Autodesk Fusion 360 part; units mm, degrees
sketch "Sketch1" plane through (0, 0, 0) normal (0, 0, 1) x (1, 0, 0)
  line L0 (0, 0) -> (20, 0)
  line L1 (20, 90) -> (0, 90)
  line L2 (0, 90) -> (0, 0)
  line L3 (4, 79) -> (11.125, 79)
  line L4 (11.125, 79) -> (11.125, 84)
  line L5 (4, 11) -> (4, 79)
  line L6 (0, 75) -> (0, 25)
  line L7 (20, 90) -> (0, 0) construction
  line L8 (0, 90) -> (20, 0) construction
  line L9 (0, 90) -> (-23, 90)
  line L10 (-23, 90) -> (-23, 0)
  line L11 (-23, 0) -> (0, 0)
  line L12 (0, 0) -> (0, 90)
  line L13 (0, 90) -> (-23, 0) construction
  line L14 (-23, 90) -> (0, 0) construction
  line L15 (10, 45) -> (-11.5, 45) construction
  line L16 (0, 86) -> (-19, 86)
  line L17 (-19, 86) -> (-19, 4)
  line L18 (-19, 4) -> (0, 4)
  line L19 (12, 90) -> (12, 0) construction
  line L20 (11.125, 84) -> (12, 84)
  line L21 (20, 79) -> (12.875, 79)
  line L22 (12.875, 79) -> (12.875, 84)
  line L23 (12.875, 84) -> (12, 84)
  line L24 (20, 90) -> (20, 0)
  line L25 (20, 11) -> (12.875, 11)
  line L26 (4, 11) -> (11.125, 11)
  line L27 (11.125, 11) -> (11.125, 6)
  line L28 (11.125, 6) -> (12, 6)
  line L29 (12.875, 6) -> (12, 6)
  line L30 (12.875, 11) -> (12.875, 6)
  point P0 (-11.5, 45)
  dimension "d37" = 90
  dimension "d38" = 23
  dimension "d39" = -4
  dimension "d51" = 12
  dimension "d57" = 1.75
  dimension "d63" = 5
  dimension "d65" = 78
  dimension "d66" = 6
  dimension "d67" = 20
  dimension "d72" = 8
extrude "Extrude7" add sketch "Sketch1" along normal blind 5 contours L2 L6 L12 L16 L17 L18 | L3 L4 L5 L20 L21 L22 L23 L24 L25 L26 L27 L28 L29 L30 makes body 1 at (6.375, 33.6667, 0) makes body 2 at (-6.3333, 58.6667, 0)
extrude "Extrude9" add sketch "Sketch1" along normal blind 70 contours L0 L1 L2 L3 L4 L5 L6 L12 L20 L21 L22 L23 L24 L25 L26 L27 L28 L29 L30 bodies 1 2
extrude "Extrude10" add sketch "Sketch1" along normal blind 100 contours L2 L9 L10 L11 L12 L16 L17 L18 bodies 1
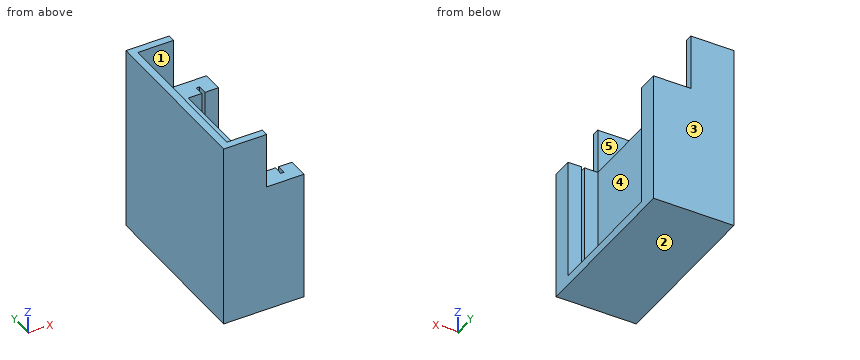
Geometry: final body of the model. Coordinates: model frame, mm. Face numbers are marked on the shaded views. A direction names the side the tool comes from. Round coordinates to 2 decimals unless told otherwise and drop trailing zeros. Loops run counter-clockwise (first coordinate to the right, second up) from the corner with the lowest first, then second, coordinate; pieces in that order, holes last. Notation, with made-up numbers: (-12.75, 59) -> (-1.75, 59) arc R30 cw to (-1.75, 90) -> close; hole circle Ø9 at (11.5, 79.5). An arc over 180 degrees is marked (long way). Use one line per item in the form item = value. Start each with the question number.
1) Section B-B on z = 72. Output: boundary loops of the cut face in (x, y), then the cut area to 3 significant figures.
2) Section A-A on z = 55. Output: boundary loops of the cut face in (x, y) (3 decimals).
3) Section C-C on y = 39.5. Output: boundary loops of the cut face in (x, z), then the cut area to 3 significant figures.
4) First-contact query: P1, Ø4, axis at x = 2.5, z = 76.5, coming from the -Y side; P2, Ø1, axis at y = 70.5, z = 73.5, coming from the +X side; P3, Ø3, axis at y = 2.5, z = 92.5, coming from the +X side; P4, Ø4, axis at y = 70, z = 26, coming from the +X side. Flat tips, straight axial feed; report the tip coordinate or a pass-through.
5) Draft query along X for the marked faces 3, 4 and 5. Return one class per face: released by +X, released by -X, zero draft, split by the parting line, or undercut.
6) Section D-D on x = -10. Output: boundary loops of the cut face in (y, z).
7) Access query for the marked faces 1 and 2. Directions: +Z, -Z, +X, -X, +Y, -Y. A direction counts if a zero-diameter tool reaches every point of the face in a straight line with its end or side. Return the directions, or none.
8) Line query: L1, parallel to X at y = 25.5, z = 60; L2, parallel to Y at x = -18, z = 63.5; L3, parallel to X at y = 7, z = 20 (3 decimals). Output: solid intervals per line, ascending.
Response:
q1.outline = (-23, 0) -> (0, 0) -> (0, 4) -> (-19, 4) -> (-19, 86) -> (0, 86) -> (0, 90) -> (-23, 90) -> close
q1.area = 512 mm^2
q2.outline = (-23, 0) -> (20, 0) -> (20, 11) -> (12.875, 11) -> (12.875, 6) -> (11.125, 6) -> (11.125, 11) -> (4, 11) -> (4, 79) -> (11.125, 79) -> (11.125, 84) -> (12.875, 84) -> (12.875, 79) -> (20, 79) -> (20, 90) -> (-23, 90) -> close; hole (-19, 4) -> (0, 4) -> (0, 86) -> (-19, 86) -> close
q3.outline = (-23, 0) -> (20, 0) -> (20, 5) -> (4, 5) -> (4, 70) -> (0, 70) -> (0, 5) -> (-19, 5) -> (-19, 100) -> (-23, 100) -> close
q3.area = 855 mm^2
q4.P1 = through
q4.P2 = -19
q4.P3 = 0
q4.P4 = 4
q5.face_3 = zero draft
q5.face_4 = released by +X
q5.face_5 = undercut
q6.outline = (0, 0) -> (90, 0) -> (90, 100) -> (86, 100) -> (86, 5) -> (4, 5) -> (4, 100) -> (0, 100) -> close
q7.face_1 = +Z
q7.face_2 = -Z, +X, -X, +Y, -Y
q8.L1 = -23 to -19, 0 to 4
q8.L2 = 0 to 4, 86 to 90
q8.L3 = -23 to -19, 0 to 11.125, 12.875 to 20
